from build123d import *

# Parameters (mm, degrees)
SKETCH_1_W      = 146.451560669
SKETCH_1_H      = 102.5
SKETCH_1_R      = 2.329290182
SKETCH_1_R_2    = 2.3
EXTRUDE_1_DEPTH = 10


with BuildPart() as part:
    # Эскиз1 → Бобышка-Вытянуть1 (new body)
    with BuildSketch(Plane(origin=(0, 236.195974268, 0), x_dir=(1, 0, 0), z_dir=(0, 1, 0))):
        with Locations((64.784761029, -89.523129836)):
            Rectangle(SKETCH_1_W, SKETCH_1_H)
        with Locations(Location((64.808980694, -43.273129836, 0), (0, 0, 180))):
            Circle(SKETCH_1_R, mode=Mode.SUBTRACT)
        with Locations(Location((-3.441019306, -89.187817333, 0), (0, 0, 180))):
            Circle(SKETCH_1_R_2, mode=Mode.SUBTRACT)
        with Locations(Location((64.808980694, -135.773129836, 0), (0, 0, 180))):
            Circle(SKETCH_1_R, mode=Mode.SUBTRACT)
        with Locations(Location((133.058980694, -89.523129836, 0), (0, 0, 180))):
            Circle(SKETCH_1_R_2, mode=Mode.SUBTRACT)
        with Locations(Location((-3.441019306, -43.273129836, 0), (0, 0, 180))):
            Circle(SKETCH_1_R_2, mode=Mode.SUBTRACT)
        with Locations(Location((133.058980694, -43.273129836, 0), (0, 0, 180))):
            Circle(SKETCH_1_R_2, mode=Mode.SUBTRACT)
        with Locations(Location((133.058980694, -135.773129836, 0), (0, 0, 180))):
            Circle(SKETCH_1_R_2, mode=Mode.SUBTRACT)
        with Locations(Location((-3.441019306, -135.773129836, 0), (0, 0, 180))):
            Circle(SKETCH_1_R_2, mode=Mode.SUBTRACT)
        Polygon((1.591962046, -130.773129836), (1.558980694, -48.273129836), (128.058980694, -48.273129836), (128.058980694, -130.773129836), align=None, mode=Mode.SUBTRACT)
    extrude(amount=EXTRUDE_1_DEPTH)


solid = part.part
Here's how the part is built. I have some questions about the finished solid (model axes, mm). A direction names the side the tool comes from. Give positions to 0.01 mm unless a question says otherwise; leave off trailing zeros. Order: outer loops, then holes, each group sorted by start corner. A loop starts at its lowest first (then second) coordinate and runs counter-clockwise, first axis right, second up. Notation, with made-up numbers: M -33,86.25 L -25,86.25 A26 ccw -25,108.25 Z; hole C 66.5,44 d4. An arc over 180 degrees is marked long. Answer as a JSON object with one key per item and string values. Group by question number.
1) I'm going to push a flat-ended pin straight in: pin 1 Ø4 at (x, z) = (64.81, 135.77) entering from -Y. Where does the tip first touch, or does it pass through?
2) We'd pull the mould along X, two halves only. Please class faces 1 (the flat face through (64, 236.196, 131)), 2 (the flat face through (138.011, 241, 90)), 3 (the flat face through (-8.441, 241, 90)), 4 (the cylindrical face through (-2.942, 241.126, 86.943)): pulls with the +X half, pulls with the -X half, needs draft (parallel to the pull), parting line crosses it, or undercut.
3) Suppose I cut it at C-C, the plane y = 244.75. Count the separate pieces of the cut face and the enclosed holes in it, plus the area to 3 significant figures.
4) Suppose I cut it at B-B, the plane z = 99. Write out the boundary of the cut face in (x, y).
5) Suppose I cut it at A-A, the plane x = 95. Write out the boundary of the cut face in (y, z), plus the area to 3 significant figures.
6) On a 3-axis mill with a long thin cutter (end or side, diameter ignored), from which of +Z, -Z, +X, -X, +Y, -Y can I reach the whole of each face in a straight line? I mean faces 5 (the flat face through (64, 246.196, 131)), 6 (the flat face through (64, 241, 48.273)). Say none if no direction works.
7) Please list where these lines run through material, in increasing order: L1, parallel to Z at x = 79, y = 242.5; L2, parallel to X at y = 243.5, z = 49.5; L3, parallel to Z at x = 65, y = 239.5. Write a range as [from, to].
Results found:
{
 "1": {"pin 1": "through"},
 "2": {"face 1": "needs draft", "face 2": "pulls with the +X half", "face 3": "pulls with the -X half", "face 4": "undercut"},
 "3": {"separate pieces": "1", "enclosed holes": "9", "area": "4,440 mm²"},
 "4": {"outline": "M -8.44,236.2 L 1.58,236.2 L 1.58,246.2 L -8.44,246.2 Z; M 128.06,236.2 L 138.01,236.2 L 138.01,246.2 L 128.06,246.2 Z"},
 "5": {"outline": "M 236.2,38.27 L 246.2,38.27 L 246.2,48.27 L 236.2,48.27 Z; M 236.2,130.77 L 246.2,130.77 L 246.2,140.77 L 236.2,140.77 Z", "area": "200 mm²"},
 "6": {"face 5": "+Z, -Z, +X, -X, +Y", "face 6": "+Y, -Y"},
 "7": {"L1": "[38.27, 48.27], [130.77, 140.77]", "L2": "[-8.44, 1.56], [128.06, 138.01]", "L3": "[38.27, 40.95], [45.59, 48.27], [130.77, 133.45], [138.09, 140.77]"}
}
